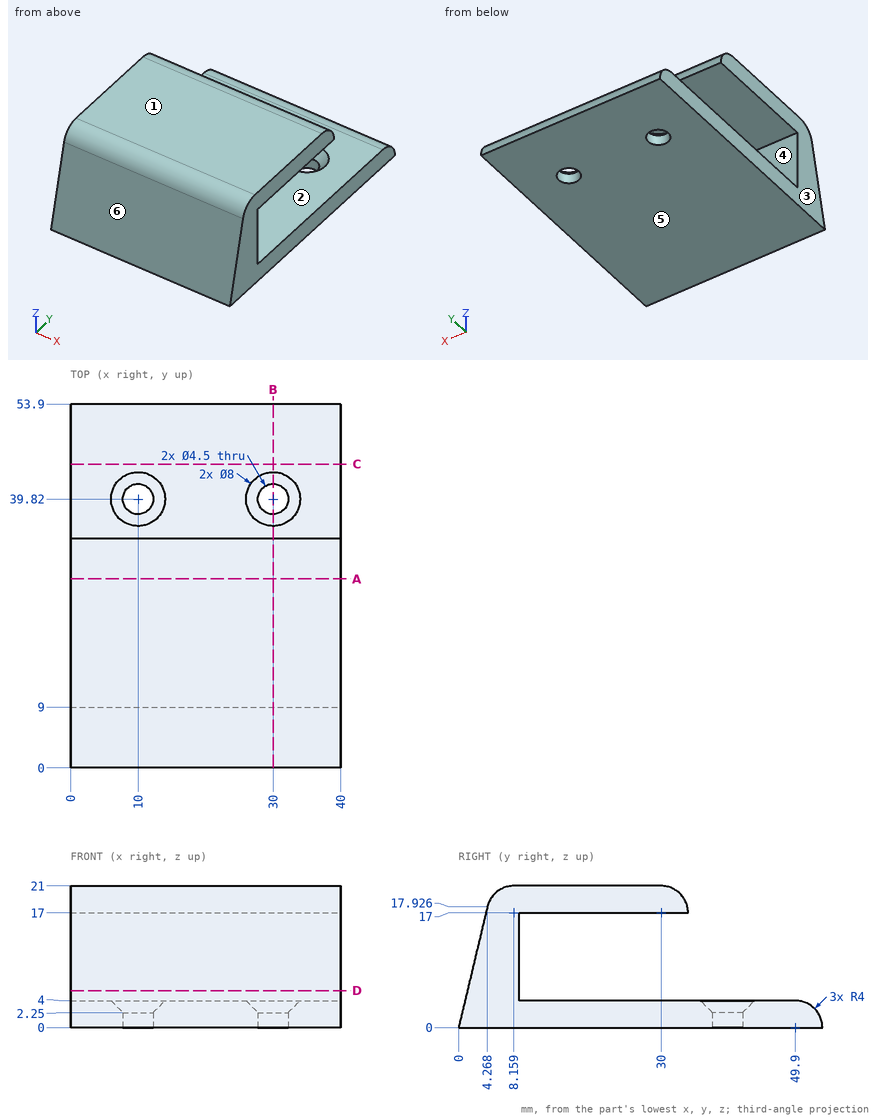
Study the drawing (mm; zero at the part's minimum x, y, z) and answer. A direction names the side the tool comes from. Coordinates: 2 decimals unless noted, no trailing zeros. Write each loop counter-clockwise with the first axis right and the second up, starting at its lowest first coordinate (ties: lowest second). Pieces come first, ordered by that corner, then holes. Notation, with made-up numbers: (6.25, -19) - (54.25, -19) arc R17 cw to (54.25, 6) - close; hole circle Ø7 at (72.5, 66.5). An arc over 180 degrees is marked (long way). Put each result on its own line as item: value.
1. The part is cut by section A-A on y = 28. Give the vertices of the cut face in (x, z), plus the area to 3 significant figures.
Answer sheet:
outline: (0, 0) - (40, 0) - (40, 4) - (0, 4) - close; (0, 17) - (40, 17) - (40, 21) - (0, 21) - close
area: 320 mm^2
2. The part is cut by section C-C on y = 45. Give the vertices of the cut face in (x, z).
Answer sheet:
outline: (0, 0) - (40, 0) - (40, 4) - (0, 4) - close
3. The part is cut by section B-B on x = 30. Give the vertices of the cut face in (y, z).
Answer sheet:
outline: (0, 0) - (37.57, 0) - (37.57, 2.25) - (35.82, 4) - (9, 4) - (9, 17) - (34, 17) arc R4 ccw to (30, 21) - (8.16, 21) arc R4 ccw to (4.27, 17.93) - close; (42.07, 0) - (53.9, 0) arc R4 ccw to (49.9, 4) - (43.82, 4) - (42.07, 2.25) - close
4. The part is cut by section D-D on z = 5.5. Give the vertices of the cut face in (x, y).
Answer sheet:
outline: (0, 1.31) - (40, 1.31) - (40, 9) - (0, 9) - close
5. Find the intervals of material crossed by line 1 along Z through (x, y) = (37, 28); line 2 along Z through (x, y) = (15, 36); line 3 along Y through (x, z) = (10, 0.5), in increasing order. Write a range as from..to.
Answer sheet:
line 1: z = 0..4, 17..21
line 2: z = 0..4
line 3: y = 0.12..37.57, 42.07..53.87
6. Flat-ended cylindrical pins translate along their axes: pin 1 Ø5 at (x, z) = (16.5, 17) entering from -Y; pin 2 Ø1 at (x, z) = (9.5, 8.5) entering from -Y (1 decimal); pin 3 Ø5 at (x, z) = (12.5, 2.5) entering from +Y; pin 4 Ø6 at (x, z) = (7, 4) entering from -Y. Find the tip coordinate at first contact, or state that the pin passes through.
Answer sheet:
pin 1: stops at y = 3.45
pin 2: stops at y = 1.9
pin 3: stops at y = 53.9
pin 4: stops at y = 0.24
7. Determine the mould class of the marked faces 3, 4, 5 and 6 for opening direction Z: pulls with the +Z half, pulls with the -Z half, needs draft (parallel to the pull), parting line crosses it, or undercut.
Answer sheet:
face 3: needs draft
face 4: undercut
face 5: pulls with the -Z half
face 6: pulls with the +Z half
8. A tool of negligible diameter and unlimited length cuts with its end or side. For the marked faces 1 and 2, from which of +Z, -Z, +X, -X, +Y, -Y can it reach the whole face along a straight path? Write none if from no direction.
Answer sheet:
face 1: +Z, +X, -X, +Y, -Y
face 2: +X, -X, +Y
